```python
from build123d import *

# Parameters (mm, degrees)
SKETCH1_W           = 6.398334728
SKETCH1_H           = 1.579308664
BOSS_EXTRUDE1_DEPTH = 1.524


with BuildPart() as part:
    # Sketch1 → Boss-Extrude1 (new body)
    with BuildSketch(Plane.XY):
        Polygon((-23.403233798, -4.133198011), (-28.761615364, -5.146272329), (-28.478498191, -6.643743753), (-31.47344104, -7.209978099), (-31.756558213, -5.712506675), (-40.495294208, -7.364682597), (-40.212177035, -8.862154021), (-43.207119883, -9.428388367), (-43.490237056, -7.930916943), (-48.355985293, -8.850852284), (-53.593355447, -8.096704042), (-53.810561584, -9.605146117), (-56.827445734, -9.170733844), (-56.610239597, -7.662291769), (-78.191926721, -4.554665056), (-78.409132858, -6.063107132), (-81.426017008, -5.628694858), (-81.208810872, -4.120252783), (-99.239134473, -1.524), (-77.300143281, -1.524), (-77.300143281, 0), (-72.220143281, 0), (-72.220143281, -1.524), (-45.797700006, -1.524), (-45.797700006, 0), (-40.717700006, 0), (-40.717700006, -1.524), (-23.943865748, -1.524), align=None)
        with Locations((-45.156817929, -4.922852343)):
            Rectangle(SKETCH1_W, SKETCH1_H, mode=Mode.SUBTRACT)
    extrude(amount=-BOSS_EXTRUDE1_DEPTH)


solid = part.part
```
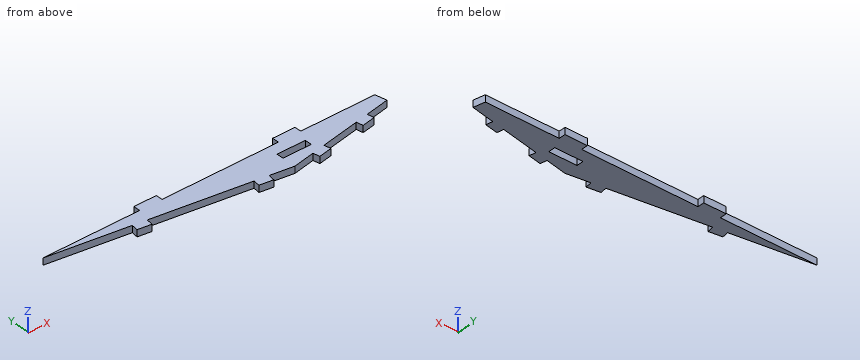
Check sheet for the modelled part. Datum: model origin and axes. Units: mm. Coordinates: 2 decimals unless noted, no trailing zeros. Loops run counter-clockwise (first coordinate to the right, second up) from the corner with the lowest first, then second, coordinate; pieces in that order, holes last. Notation, with made-up numbers: M 28,63 L 55,63 A23 ccw 55,95 Z; hole C 73.25,50 d1. An arc over 180 degrees is marked long. Answer as a JSON object with one key per item and string values.
1. Sectioned sample at C-C on y = -3.5. Record the cut outline in (x, z), and give its area (3 significant figures).
Outcome:
{"outline": "M -85.52,-1.52 L -23.53,-1.52 L -23.53,0 L -85.52,0 Z", "area": "94.5 mm²"}
2. Scan lines: L1, parallel to X at y = -1, z = -0.2; L2, parallel to Y at x = -46, z = -0.65; L3, parallel to Y at x = -55, z = -0.95. Record each from-to range of solid material in increasing order. Write a range as from..to.
Outcome:
{"L1": "-77.3..-72.22, -45.8..-40.72", "L2": "-8.41..-5.71, -4.13..-1.52", "L3": "-9.43..-1.52"}
3. Sectioned sample at B-B on x = -49.5. Record the cut outline in (y, z).
Outcome:
{"outline": "M -8.69,-1.52 L -1.52,-1.52 L -1.52,0 L -8.69,0 Z"}
4. Depth check by flat-ended pin: P1, Ø0.8, axis at y = -1, z = -0.5, coming from the -X side; P2, Ø0.5, axis at x = -44, z = -0.5, coming from the +Y side; P3, Ø0.8, axis at x = -54, z = -1, coming from the +Y side; P4, Ø0.8, axis at x = -44.5, z = -0.5, coming from the -Y side. Enter the tip coordinate at first touch or a pass-through.
Outcome:
{"P1": "x = -77.3", "P2": "y = 0", "P3": "y = -1.52", "P4": "y = -8.2"}
